from build123d import *

# Parameters (mm, degrees)
F0_R     = 57.15
F1_DEPTH = 31.75
F2_T     = -5.08
F4_W     = 25.4
F4_H     = 25.4
F5_DEPTH = 19.05
F6_R     = 2.53999
F7_R     = 9.525
F8_DEPTH = 15.875
F9_SIZE  = 1.905


# Not quite as in the source:
# - a fillet or chamfer is up to 0.001 mm smaller than in the source, because OpenCascade refuses the exact size


with BuildPart() as f1:
    # F0 (on Front) → F1 (new body)
    with BuildSketch(Plane.XZ):
        Circle(F0_R)
    extrude(amount=F1_DEPTH)

    # F2
    f2_openings = [f1.faces().sort_by_distance(p)[0] for p in [
        (0, -31.75, 0),
    ]]
    offset(amount=F2_T, openings=f2_openings)

    # F4 (on offset) → F5 (join)
    with BuildSketch(Plane.XY.offset(-50.8)):
        with Locations((0, -15.875)):
            Rectangle(F4_W, F4_H)
    extrude(amount=-F5_DEPTH)

    # F6 (radius 2.54 in the source; OpenCascade refuses exactly that, so slightly less here)
    f6_edges = [f1.edges().sort_by_distance(p)[0] for p in [
        (-57.15, -31.75, 0),
        (-52.07, -31.75, 0),
        (-57.15, 0, 0),
    ]]
    fillet(f6_edges, radius=F6_R)

    # F7 (on face) → F8 (join)
    with BuildSketch(Plane(origin=(0, 0, -69.85), x_dir=(1, 0, 0), z_dir=(0, 0, -1))):
        with Locations((0, 15.875)):
            Circle(F7_R)
    extrude(amount=F8_DEPTH)

    # F9
    f9_edges = [f1.edges().sort_by_distance(p)[0] for p in [
        (-9.525, -15.875, -85.725),
    ]]
    chamfer(f9_edges, length=F9_SIZE)


solid = f1.part
Verification items for the finished model (mm, model axes). A direction names the side the tool comes from. Coordinates: 2 decimals unless noted, no trailing zeros. One line per question, with ' | ' between items.
1) Material ranges on L1, parallel to Z at x = 0, y = -16 (3 decimals); L2, parallel to Y at x = -43, z = 9; L3, parallel to X at y = -26.5, z = -37, recorded low to high.
Solutions:
L1: -85.725 to -50.8, 52.07 to 57.15 | L2: -5.08 to 0 | L3: -43.56 to -36.64, 36.64 to 43.56
2) Depth check by flat-ended pin: pin 1 Ø6 at (x, z) = (10, -71) entering from -Y (3 decimals); pin 2 Ø4 at (x, y) = (-15.5, -13) entering from -Z; pin 3 Ø1 at (x, z) = (-33.5, -27.5) entering from +Y; pin 4 Ø12 at (x, y) = (-18, -19.5) entering from -Z. Enter the tip coordinate at first touch or a pass-through.
Solutions:
pin 1: y = -28.575 | pin 2: z = -55.53 | pin 3: y = 0 | pin 4: z = -69.85
3) Access from +Z, -Z, +X, -X, +Y, -Y to the whole of each face (thin tool, end or side, straight path). Record for faces 1 (the face through (-1, -5.08, 1)), 2 (the face through (-1.24, -25.32, -76.74)), 3 (the face through (12.7, -16, -63)).
Solutions:
face 1: -Y | face 2: -Z | face 3: -Z, +X, +Y, -Y
4) Release check for a two-part mould opening along Z. For faces 4 (the face through (0, -17, -50.8)), 5 (the face through (28, -17, 43.9)), 6 (the face through (-7.44, -15.688, 56.664)), 7 (the face through (5, -7, -69.85)) record: +Z half, -Z half, draft (parallel to the pull), parting line (faces both ways), or undercut.
Solutions:
face 4: undercut | face 5: undercut | face 6: parting line | face 7: -Z half
